Check sheet for the modelled part. Datum: model origin and axes. Units: mm. Give positions to 0.01 mm unless a question says otherwise; leave off trailing zeros. Order: outer loops, then holes, each group sorted by start corner. A loop starts at its lowest first (then second) coordinate and runs counter-clockwise, first axis right, second up.
Item 1: Sectioned sample at B-B on z = -108. Record the boundary of the cut face in (x, y), and give its area (3 significant figures).
Item 2: Gauge pin test, flat end, axial feed: P1, Ø1, axis at x = 61.5, y = 2, coming from the -Z side. Record the tip position at first contact, or that the pin passes through.
Item 3: Sectioned sample at A-A on z = -88. Record the boundary of the cut face in (x, y), and give its area (3 significant figures).
Item 4: Sectioned sample at C-C on y = 3.9. Count the separate pieces of the cut face and the enclosed holes in it, and give its area (3 significant figures).
Item 5: Sectioned sample at D-D on x = 6.5. Record the boundary of the cut face in (y, z).
Item 6: Material ranges on line 1 along X through (y, z) = (0.3, -24); line 2 along Z through (x, y) = (116, 1.15); line 3 along X through (y, z) = (1.2, -6.5), recorded low to high.
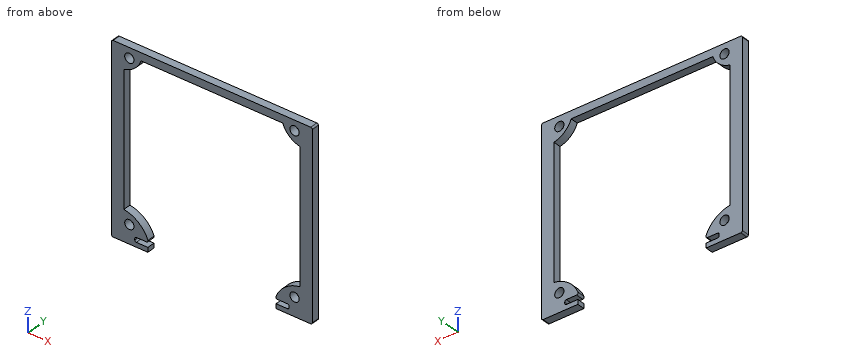
from build123d import *

# Parameters (mm, degrees)
SKETCH1_W           = 130
SKETCH1_H           = 120
SKETCH1_R           = 3
BOSS_EXTRUDE1_DEPTH = 5
SKETCH2_W           = 100
SKETCH2_H           = 3
CUT_EXTRUDE1_DEPTH  = 10
FILLET1_R           = 1
FILLET2_R           = 1
FILLET3_R           = 1
SKETCH3_W           = 83.01861615
SKETCH3_H           = 6.438048513
CUT_EXTRUDE2_DEPTH  = 10
SKETCH4_W           = 3
SKETCH4_H           = 92.008130055
BOSS_EXTRUDE2_DEPTH = 5
FILLET4_R           = 1


with BuildPart() as part:
    # Sketch1 → Boss-Extrude1 (new body)
    with BuildSketch(Plane(origin=(0, 0, 0), x_dir=(1, 0, 0), z_dir=(0, 1, 0))):
        with Locations((60, 60)):
            Rectangle(SKETCH1_W, SKETCH1_H)
        with Locations(Location((6.5, 6.5, 0), (0, 0, 270))):
            Circle(SKETCH1_R, mode=Mode.SUBTRACT)
        with Locations(Location((113.5, 6.5, 0), (0, 0, 270))):
            Circle(SKETCH1_R, mode=Mode.SUBTRACT)
        with Locations(Location((6.5, 108, 0), (0, 0, 270))):
            Circle(SKETCH1_R, mode=Mode.SUBTRACT)
        with Locations(Location((113.5, 108, 0), (0, 0, 270))):
            Circle(SKETCH1_R, mode=Mode.SUBTRACT)
        with BuildLine():
            Line((0, 100), (0, 15))
            ThreePointArc((0, 15), (8.660254038, 12.247448714), (14.142135624, 5))
            Line((14.142135624, 5), (15, 5))
            Line((15, 5), (105, 5))
            Line((105, 5), (105.857864376, 5))
            ThreePointArc((105.857864376, 5), (111.339745962, 12.247448714), (120, 15))
            Line((120, 15), (120, 100))
            ThreePointArc((120, 100), (107.752551286, 104.188611699), (100.635083269, 115))
            Line((100.635083269, 115), (100, 115))
            Line((100, 115), (20, 115))
            Line((20, 115), (19.364916731, 115))
            ThreePointArc((19.364916731, 115), (12.247448714, 104.188611699), (0, 100))
        make_face(mode=Mode.SUBTRACT)
    extrude(amount=BOSS_EXTRUDE1_DEPTH)

    # Sketch2 → Cut-Extrude1 (cut)
    with BuildSketch(Plane(origin=(0, 5, 0), x_dir=(1, 0, 0), z_dir=(0, 1, 0))):
        with Locations((60, 115.5)):
            Rectangle(SKETCH2_W, SKETCH2_H)
    extrude(amount=-CUT_EXTRUDE1_DEPTH, mode=Mode.SUBTRACT)

    # Fillet1
    fillet1_edges = [part.edges().sort_by_distance(p)[0] for p in [
        (10, 2.5, -114),
        (10, 2.5, -117),
        (110, 2.5, -117),
        (110, 2.5, -114),
    ]]
    fillet(fillet1_edges, radius=FILLET1_R)

    # Fillet2
    fillet2_edges = [part.edges().sort_by_distance(p)[0] for p in [
        (19.078784028, 2.5, -114),
    ]]
    fillet(fillet2_edges, radius=FILLET2_R)

    # Fillet3
    fillet3_edges = [part.edges().sort_by_distance(p)[0] for p in [
        (100.921215972, 2.5, -114),
    ]]
    fillet(fillet3_edges, radius=FILLET3_R)

    # Sketch3 → Cut-Extrude2 (cut)
    with BuildSketch(Plane(origin=(0, 5, 0), x_dir=(1, 0, 0), z_dir=(0, 1, 0))):
        with Locations((60, 116.780975744)):
            Rectangle(SKETCH3_W, SKETCH3_H)
    extrude(amount=-CUT_EXTRUDE2_DEPTH, mode=Mode.SUBTRACT)

    # Sketch4 → Boss-Extrude2 (add)
    with BuildSketch(Plane(origin=(0, 5, 0), x_dir=(1, 0, 0), z_dir=(0, 1, 0))):
        with Locations((118.5, 57.563435723)):
            Rectangle(SKETCH4_W, SKETCH4_H)
        with Locations((1.479834165, 57.563435723)):
            Rectangle(SKETCH4_W, SKETCH4_H)
    extrude(amount=-BOSS_EXTRUDE2_DEPTH)

    # Fillet4
    fillet4_edges = [part.edges().sort_by_distance(p)[0] for p in [
        (125, 2.5, -120),
        (125, 2.5, 0),
        (-5, 2.5, 0),
        (-5, 2.5, -120),
    ]]
    fillet(fillet4_edges, radius=FILLET4_R)


solid = part.part
Report:
1. outline: (-5, 0) - (3.5, 0) - (3.5, 5) - (-5, 5) - close; (9.5, 0) - (16, 0) - (16, 5) - (9.5, 5) - close; (104, 0) - (110.5, 0) - (110.5, 5) - (104, 5) - close; (116.5, 0) - (125, 0) - (125, 5) - (116.5, 5) - close
1. area: 150 mm2
2. P1: stops at z = -5
3. outline: (-5, 0) - (2.98, 0) - (2.98, 5) - (-5, 5) - close; (117, 0) - (125, 0) - (125, 5) - (117, 5) - close
3. area: 79.9 mm2
4. separate pieces: 1
4. enclosed holes: 4
4. area: 2,960 mm2
5. outline: (0, -120) - (5, -120) - (5, -111) - (0, -111) - close; (0, -105) - (5, -105) - (5, -101.09) - (0, -101.09) - close; (0, -13.52) - (5, -13.52) - (5, -9.5) - (0, -9.5) - close; (0, -3.5) - (5, -3.5) - (5, 0) - (0, 0) - close
6. line 1: x = -5 to 2.98, 117 to 125
6. line 2: z = -120 to -109.66, -106.34 to -100.4, -14.46 to -8.16, -4.84 to 0
6. line 3: x = -5 to 3.5, 9.5 to 13.52, 106.48 to 110.5, 116.5 to 125
